The model under review builds one solid part; all positions refer to its coordinate system, in mm. Face numbers are marked on the shaded views. A direction names the side the tool comes from. Give positions to 0.01 mm unless a question says otherwise; leave off trailing zeros. Loops run counter-clockwise (first coordinate to the right, second up) from the corner with the lowest first, then second, coordinate; pieces in that order, holes last. Notation, with made-up numbers: (77.5, 55) - (108.5, 55) arc R16 ccw to (108.5, 68) - close; hole circle Ø11 at (-9, -10.75). An arc over 180 degrees is marked (long way). Return JSON: item names as keys, results as strings. Group by question number.
from build123d import *

# Parameters (mm, degrees)
F0_W      = 28.971875
F0_H      = 28.971875
F0_W_2    = 25.796875
F0_H_2    = 25.796875
F1_DEPTH  = 14.2875
F2_W      = 25.796875
F2_H      = 25.796875
F3_DEPTH  = 1.5875
F6_DEPTH  = 3.175
F8_R      = 1.5875
F9_DEPTH  = 1.5885
F10_W     = 12.7
F10_H     = 3.175
F11_DEPTH = 1.5875


# Not quite as in the source:
# - a pattern or mirror of a feature is missing from the dataset's text; its kind, count and spacing are read off the source's solid


with BuildPart() as f1:
    # F0 (on Top) → F1 (new body)
    with BuildSketch(Plane.XY):
        Rectangle(F0_W, F0_H)
        Rectangle(F0_W_2, F0_H_2, mode=Mode.SUBTRACT)
    extrude(amount=F1_DEPTH)

    # F2 (on face) → F3 (join)
    with BuildSketch(Plane(origin=(0, 0, 0), x_dir=(1, 0, 0), z_dir=(0, 0, -1))):
        Rectangle(F2_W, F2_H)
    extrude(amount=-F3_DEPTH)

    # F4: union 

    # F5 (on Front) → F6 (join, symmetric)
    with BuildSketch(Plane.XZ):
        Polygon((14.4859375, 11.90625), (14.4859375, 10.31875), (15.6765625, 10.6377770072), align=None)
    f6 = extrude(amount=F6_DEPTH, both=True)

    # F6_copies: F6 across plane
    add(f6.mirror(Plane(origin=(0, 0, 0), x_dir=(0, 0, -1), z_dir=(-1, 0, 0))))

    # F8 (on face) → F9 (cut, through all)
    with BuildSketch(Plane.XY.offset(1.5875)):
        with Locations((0, 6.35)):
            Circle(F8_R)
        with Locations((0, -6.35)):
            Circle(F8_R)
    extrude(amount=-F9_DEPTH, mode=Mode.SUBTRACT)

    # F10 (on face) → F11 (cut, through all)
    with BuildSketch(Plane.XZ.offset(14.4859375)):
        with Locations((0, 6.35)):
            Rectangle(F10_W, F10_H)
    extrude(amount=-F11_DEPTH, mode=Mode.SUBTRACT)


solid = f1.part
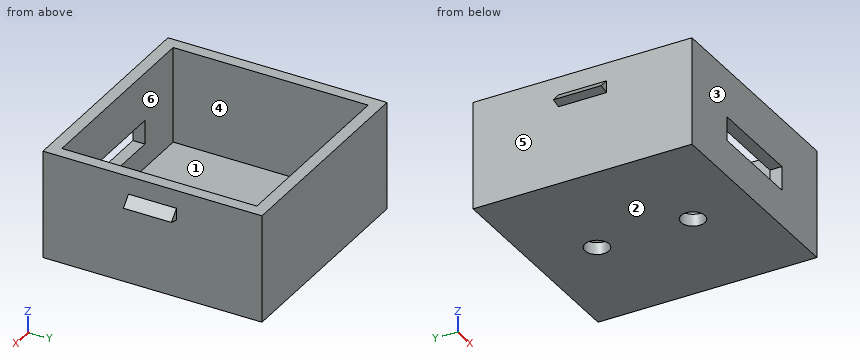
Item 1: For P1, Ø4.5, axis at y = -1, z = 7, coming from the -X side; P2, Ø7, axis at y = 2, z = 4.5, coming from the +X side; P3, Ø4, axis at x = 9.5, y = -2.5, coming from the +Z side; P4, Ø3, axis at x = 0, y = -6.35, coming from the +Z side, all flat-tipped, find the tip position at first contact; note any pin that passes through.
Item 2: Take a section at B-B (y = 6.35). State the section outline as (x, z) points, then the cut area to 3 significant figures.
Item 3: Take a section at A-A (x = 5). State the section outline as (y, z) points.
Item 4: Mouldability with a two-part tool opening along Y and no side actions: class the marked faces 3, 4, 5 and 6 as +Y half, -Y half, draft (parallel to the pull), parting line (faces both ways), or undercut.
Item 5: Take a section at C-C (z = 3.75). State the section outline as (x, y) points.
Item 6: Take a section at D-D (x = 0). State the section outline as (y, z) points, then the cut area to 3 significant figures.
Item 7: Tool access review of the marked faces 1 and 2: name each direction out of +Z, -Z, +X, -X, +Y, -Y from which nothing blocks a thin tool from reaching the whole face with its end or side.
Item 8: For L1, parallel to Y at x = 0, z = 0.9; L2, parallel to Y at x = -9.5, z = 5, list the stretches that pass through material, from the lowest coordinate up. Write a range as from..to.
Check sheet entries:
{
 "1": {"P1": "stops at x = -14.49", "P2": "stops at x = 14.49", "P3": "stops at z = 1.59", "P4": "passes through"},
 "2": {"outline": "(-14.49, 0) - (-1.59, 0) - (-1.59, 1.59) - (-12.9, 1.59) - (-12.9, 14.29) - (-14.49, 14.29) - close; (1.59, 0) - (14.49, 0) - (14.49, 14.29) - (12.9, 14.29) - (12.9, 1.59) - (1.59, 1.59) - close", "area": "81.3 mm^2"},
 "3": {"outline": "(-14.49, 0) - (14.49, 0) - (14.49, 14.29) - (12.9, 14.29) - (12.9, 1.59) - (-12.9, 1.59) - (-12.9, 4.76) - (-14.49, 4.76) - close; (-14.49, 7.94) - (-12.9, 7.94) - (-12.9, 14.29) - (-14.49, 14.29) - close"},
 "4": {"face 3": "-Y half", "face 4": "undercut", "face 5": "draft", "face 6": "undercut"},
 "5": {"outline": "(-14.49, -14.49) - (14.49, -14.49) - (14.49, 14.49) - (-14.49, 14.49) - close; hole (-12.9, -12.9) - (12.9, -12.9) - (12.9, 12.9) - (-12.9, 12.9) - close"},
 "6": {"outline": "(-14.49, 0) - (-7.94, 0) - (-7.94, 1.59) - (-12.9, 1.59) - (-12.9, 4.76) - (-14.49, 4.76) - close; (-14.49, 7.94) - (-12.9, 7.94) - (-12.9, 14.29) - (-14.49, 14.29) - close; (-4.76, 0) - (4.76, 0) - (4.76, 1.59) - (-4.76, 1.59) - close; (7.94, 0) - (14.49, 0) - (14.49, 14.29) - (12.9, 14.29) - (12.9, 1.59) - (7.94, 1.59) - close", "area": "71.2 mm^2"},
 "7": {"face 1": "+Z", "face 2": "-Z, +X, -X, +Y, -Y"},
 "8": {"L1": "y = -14.49..-7.94, -4.76..4.76, 7.94..14.49", "L2": "y = -14.49..-12.9, 12.9..14.49"}
}
